Geometry: final body of the model. Coordinates: model frame, mm. A direction names the side the tool comes from. Give positions to 0.01 mm unless a question says otherwise; leave off trailing zeros. Write each loop counter-clockwise with the first axis right and the second up, starting at its lowest first coordinate (ties: lowest second). Pieces come first, ordered by that corner, then holes. Notation, with made-up numbers: (39.5, -33) -> (84.5, -33) arc R10 ccw to (84.5, -25) -> close; hole circle Ø2 at (-36.5, -9.5). An arc over 180 degrees is marked (long way). Use CSV: the item, a comma, the result in double quotes. Start each with the question number.
1) Set-up query: faces 1 (the face through (3.07, -6.12, 14.48)), 2 (the face through (-46, -18.05, 8)), 3 (the face through (-52, -27, 3)), 4 (the face through (53, 28, 3)). Return all of +Z, -Z, +X, -X, +Y, -Y with unobstructed straight access to the full face (end or side cutting, diameter ignored); none if empty.
2) Section D-D (x = -44.5). Output: boundary loops of the cut face in (y, z).
3) Section A-A (x = 50). Output: boundary loops of the cut face in (y, z).
4) Material intervals for line 1 (Y direction, x = -50, z = 2.45); line 2 (Y direction, x = 50, z = 0.85); line 3 (Y direction, x = -32, z = 6), sorted ascending. Write a range as [from, to].
5) Draft query along X for faces 5 (the face through (-37, -32, 10)), 6 (the face through (-33, -30.05, 11)), 7 (the face through (-1.417, 2.118, 11.479)). Return one class per face: pulls with the +X half, pulls with the -X half, needs draft (parallel to the pull), parting line crosses it, or undercut.
6) Contact query for flat-ended pins moving along their axis: P1, Ø6, axis at x = 10, y = -9, coming from the -Z side; P2, Ø5, axis at x = 33.5, z = 10, coming from the -Y side (3 decimals); P3, Ø2, axis at y = -32.5, z = 8.5, coming from the -X side; P4, Ø1.2, axis at y = 24, z = 9.5, coming from the +X side. Output: stop coordinate, or through.
```python
from build123d import *

# Parameters (mm, degrees)
SKETCH_10_R     = 1.65
EXTRUDE_1_DEPTH = 3
EXTRUDE_START   = 3
EXTRUDE_2_DEPTH = 7
EXTRUDE_3_DEPTH = 13
CHAMFER_1_SIZE  = 7
EXTRUDE_5_DEPTH = 10
FILLET_1_R      = 1


with BuildPart() as part:
    # 草图10 → 凸台-拉伸1 (new body)
    with BuildSketch(Plane.XY):
        Polygon((-60, -18.05), (-31.485028843, -18.05), (23.614971157, 37.05), (60, 37.05), (60, 18.05), (31.485028843, 18.05), (-23.614971157, -37.05), (-60, -37.05), align=None)
        with Locations((-50, -27.55)):
            Circle(SKETCH_10_R, mode=Mode.SUBTRACT)
        with Locations((50, 27.55)):
            Circle(SKETCH_10_R, mode=Mode.SUBTRACT)
    extrude(amount=EXTRUDE_1_DEPTH)

    # 草图11 → 凸台-拉伸2 (add)
    with BuildSketch(Plane.XY.offset(EXTRUDE_START)):
        Polygon((-41, -18.05), (-41, -37.05), (-23.614971157, -37.05), (31.485028843, 18.05), (41, 18.05), (41, 37.05), (23.614971157, 37.05), (-31.485028843, -18.05), align=None)
    extrude(amount=EXTRUDE_2_DEPTH)

    # 草图12 → 凸台-拉伸3 (add)
    with BuildSketch(Plane.XY.offset(EXTRUDE_START)):
        Polygon((-60, -18.05), (-31.485028843, -18.05), (23.614971157, 37.05), (60, 37.05), (60, 34.05), (24.857611845, 34.05), (-30.242388155, -21.05), (-60, -21.05), align=None)
        Polygon((-60, -34.05), (-60, -37.05), (-23.614971157, -37.05), (31.485028843, 18.05), (60, 18.05), (60, 21.05), (30.242388155, 21.05), (-24.857611845, -34.05), align=None)
    extrude(amount=EXTRUDE_3_DEPTH)

    # 倒角1
    chamfer_1_edges = [part.edges().sort_by_distance(p)[0] for p in [
        (41, 27.55, 10),
        (-41, -27.55, 10),
    ]]
    chamfer(chamfer_1_edges, length=CHAMFER_1_SIZE - 0.0001)  # a hair under: the kernel refuses the full size

    # 草图15 → 凸台-拉伸5 (add)
    with BuildSketch(Plane.XY.offset(3)):
        Polygon((-37, -21.05), (-37, -25.05), (-28.585533906, -25.05), (26.514466094, 30.05), (37, 30.05), (37, 34.05), (24.857611845, 34.05), (-30.242388155, -21.05), align=None)
        Polygon((-37, -30.05), (-37, -34.05), (-24.857611845, -34.05), (30.242388155, 21.05), (37, 21.05), (37, 25.05), (28.585533906, 25.05), (-26.514466094, -30.05), align=None)
    extrude(amount=EXTRUDE_5_DEPTH)

    # 圆角1
    fillet_1_edges = [part.edges().sort_by_distance(p)[0] for p in [
        (-31.485028843, -18.05, 8),
        (23.614971157, 37.05, 8),
        (31.485028843, 18.05, 8),
        (-23.614971157, -37.05, 8),
        (-28.585533906, -25.05, 11.5),
        (26.514466094, 30.05, 11.5),
        (-26.514466094, -30.05, 11.5),
        (28.585533906, 25.05, 11.5),
        (24.857611845, 34.05, 14.5),
        (-30.242388155, -21.05, 14.5),
        (-24.857611845, -34.05, 14.5),
        (30.242388155, 21.05, 14.5),
    ]]
    fillet(fillet_1_edges, radius=FILLET_1_R)


solid = part.part
```
Answers follow:
1,face 1,"+Z"
1,face 2,"+Z, -Z, -X, +Y"
1,face 3,"+Z, -X"
1,face 4,"+Z, +X"
2,outline,"(-37.05, 0) -> (-18.05, 0) -> (-18.05, 16) -> (-21.05, 16) -> (-21.05, 3) -> (-34.05, 3) -> (-34.05, 16) -> (-37.05, 16) -> close"
3,outline,"(18.05, 0) -> (25.9, 0) -> (25.9, 3) -> (21.05, 3) -> (21.05, 16) -> (18.05, 16) -> close; (29.2, 0) -> (37.05, 0) -> (37.05, 16) -> (34.05, 16) -> (34.05, 3) -> (29.2, 3) -> close"
4,line 1,"y = [-37.05, -29.2], [-25.9, -18.05]"
4,line 2,"y = [18.05, 25.9], [29.2, 37.05]"
4,line 3,"y = [-37.05, -18.05]"
5,face 5,"pulls with the -X half"
5,face 6,"needs draft"
5,face 7,"undercut"
6,P1,"passes through"
6,P2,"stops at y = 17.565"
6,P3,"stops at x = -37"
6,P4,"stops at x = 37"
